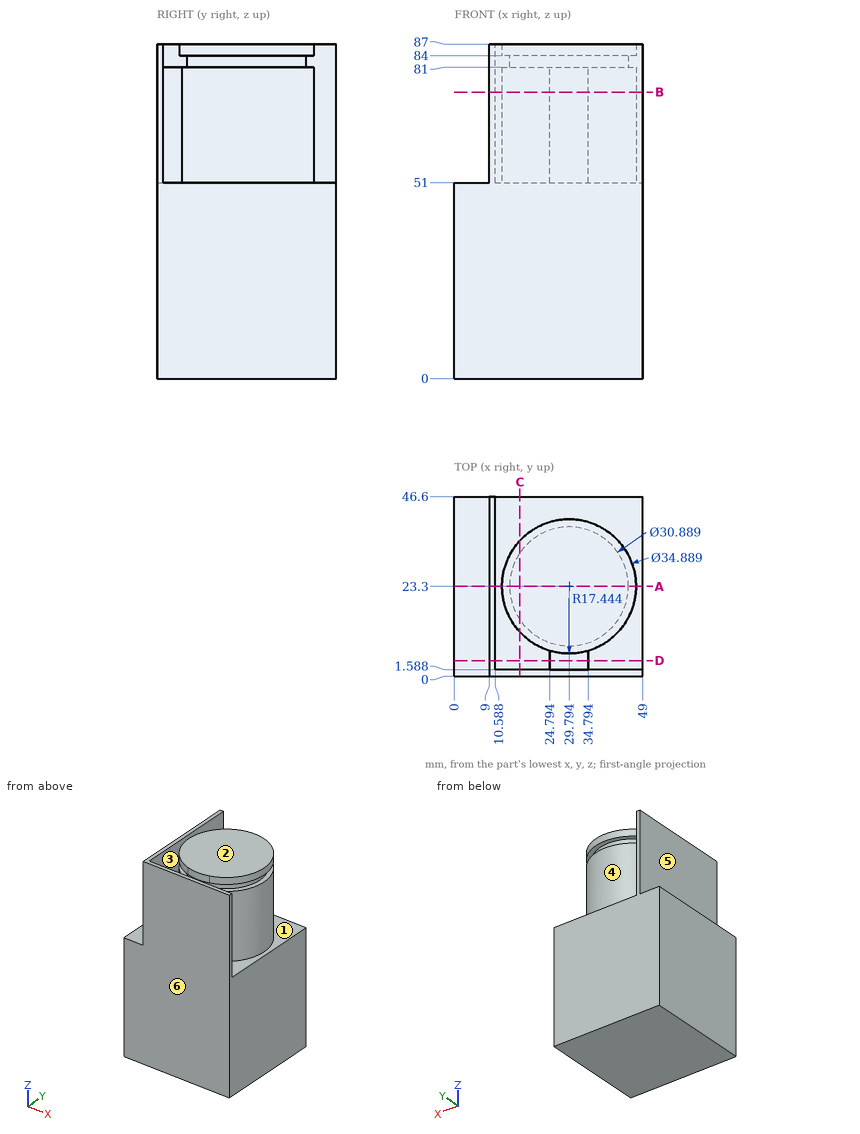
Design review of the part shown in the three views and the two pictorial views. Dimensions are in mm from the part's minimum x, y and z. A direction names the side the tool comes from. Give positions to 0.01 mm unless a question says otherwise; leave off trailing zeros. Write each loop counter-clockwise with the first axis right and the second up, starting at its lowest first coordinate (ties: lowest second). Pieces come first, ordered by that corner, then holes. Notation, with made-up numbers: M -32,75.25 L -9,75.25 A21 cw -9,112.25 Z; hole C 80.5,-9.5 d6. An arc over 180 degrees is marked long. Return JSON: item names as keys, results as strings. Group by question number.
Item 1: Wall thickness on line 1 along X through (y, z) = (5.5, 73); line 2 along Z through (x, y) = (3, 41.5); line 3 along Z through (x, y) = (33, 6): over which ranges is each line inside the solid? List them lowest first.
Item 2: Take a section at C-C (x = 17). Give the boundary of the cut face in (y, z), plus the area to 3 significant figures.
Item 3: Clearance check with flat-ended pins moving along their axes: pin 1 Ø10 at (y, z) = (39, 57.5) entering from -X; pin 2 Ø11 at (y, z) = (31, 73.5) entering from +X; pin 3 Ø1 at (x, y) = (43.5, 10) entering from +Z; pin 4 Ø12 at (x, y) = (18, 25) entering from -Z. State where each tip first meets the part, or that it passes through.
Item 4: Tool access review of the marked faces 1, 2 and 3: name each direction out of +Z, -Z, +X, -X, +Y, -Y from which nothing blocks a thin tool from reaching the whole face with its end or side.
Item 5: The part is to be moulded in two halves that separate along Y. For the marked faces 4, 5 and 6, say which applies: pulls with the +Y half, pulls with the -Y half, needs draft (parallel to the pull), parting line crosses it, or undercut.
Item 6: Take a section at A-A (y = 23.3). Give the boundary of the cut face in (x, z), plus the area to 3 significant figures.
Item 7: Take a section at D-D (y = 4). Give the boundary of the cut face in (x, z), plus the area to 3 significant figures.
Item 8: Take a section at B-B (z = 74.5). Give the boundary of the cut face in (x, y) (1 decimal).
Return value:
{
 "1": {"line 1": "x = 9 to 10.59, 24.79 to 34.79", "line 2": "z = 0 to 51", "line 3": "z = 0 to 81"},
 "2": {"outline": "M 0,0 L 46.6,0 L 46.6,51 L 35.16,51 L 35.16,81 L 31.95,81 L 31.95,84 L 35.16,84 L 35.16,87 L 11.44,87 L 11.44,84 L 14.65,84 L 14.65,81 L 11.44,81 L 11.44,51 L 1.59,51 L 1.59,87 L 0,87 Z", "area": "3,270 mm2"},
 "3": {"pin 1": "stops at x = 9", "pin 2": "stops at x = 47.1", "pin 3": "stops at z = 51", "pin 4": "stops at z = 0"},
 "4": {"face 1": "+Z", "face 2": "+Z, +X, -X, +Y, -Y", "face 3": "+Z, +Y"},
 "5": {"face 4": "undercut", "face 5": "needs draft", "face 6": "pulls with the -Y half"},
 "6": {"outline": "M 0,0 L 49,0 L 49,51 L 47.24,51 L 47.24,81 L 45.24,81 L 45.24,84 L 47.24,84 L 47.24,87 L 12.35,87 L 12.35,84 L 14.35,84 L 14.35,81 L 12.35,81 L 12.35,51 L 10.59,51 L 10.59,87 L 9,87 L 9,51 L 0,51 Z", "area": "3,800 mm2"},
 "7": {"outline": "M 0,0 L 49,0 L 49,51 L 34.79,51 L 34.79,81 L 24.79,81 L 24.79,51 L 10.59,51 L 10.59,87 L 9,87 L 9,51 L 0,51 Z", "area": "2,860 mm2"},
 "8": {"outline": "M 9,0 L 49,0 L 49,1.6 L 34.8,1.6 L 34.8,6.6 A17.4 ccw long 24.8,6.6 L 24.8,1.6 L 10.6,1.6 L 10.6,46.6 L 9,46.6 Z"}
}
